Input: part model. Units: mm. Frame: model coordinates. A direction names the side the tool comes from. Give positions to 0.01 mm unless a question says otherwise; leave off trailing zeros. Loops run counter-clockwise (first coordinate to the right, second up) from the corner with the lowest first, then second, coordinate; pieces in that order, holes last. Notation, with made-up numbers: M -37.75,27.5 L -16.75,27.5 A21 cw -16.75,44.5 Z; hole C 27,85 d4. An arc over 180 degrees is marked long. Return JSON: item names as keys, results as strings. Group by question number.
```python
from build123d import *

# Parameters (mm, degrees)
F0_W      = 76.2
F0_H      = 76.2
F1_DEPTH  = 76.2
F3_D      = 25.4
F4_W      = 25.4
F4_H      = 25.4
F5_DEPTH  = 12.7
F6_R      = 12.7
F7_DEPTH  = 12.7
F8_R      = 12.7
F9_R      = 12.7
F10_SIZE  = 5.08
F11_SIZE  = 5.08
F12_R     = 5.08
F14_DEPTH = 7.62
F16_DEPTH = 7.62
F18_DEPTH = 7.62
F20_DEPTH = 7.62
F22_DEPTH = 7.62
F24_DEPTH = 7.62


with BuildPart() as f1:
    # F0 (on Front) → F1 (new body)
    with BuildSketch(Plane.XZ):
        with Locations((38.1, 38.1)):
            Rectangle(F0_W, F0_H)
    extrude(amount=F1_DEPTH)

    # F3 (through all)
    with Locations(Plane.XY.offset(76.2)):
        with Locations((37.350509, -33.948544)):
            Hole(F3_D / 2)

    # F4 (on face) → F5 (join)
    with BuildSketch(Plane.XZ.offset(76.2)):
        with Locations((38.1, 38.1)):
            Rectangle(F4_W, F4_H)
    extrude(amount=F5_DEPTH)

    # F6 (on face) → F7 (join)
    with BuildSketch(Plane.YZ.offset(76.2)):
        with Locations((-34.955569, 38.1)):
            Circle(F6_R)
    extrude(amount=F7_DEPTH)

    # F8
    f8_edges = [f1.edges().sort_by_distance(p)[0] for p in [
        (0, -38.1, 76.2),
    ]]
    fillet(f8_edges, radius=F8_R)

    # F9
    f9_edges = [f1.edges().sort_by_distance(p)[0] for p in [
        (76.2, -38.1, 76.2),
    ]]
    fillet(f9_edges, radius=F9_R)

    # F10
    f10_edges = [f1.edges().sort_by_distance(p)[0] for p in [
        (0, -76.2, 31.75),
    ]]
    chamfer(f10_edges, length=F10_SIZE)

    # F11
    f11_edges = [f1.edges().sort_by_distance(p)[0] for p in [
        (82.55, -22.255569, 38.1),
        (76.2, -47.655569, 38.1),
        (88.9, -47.655569, 38.1),
    ]]
    chamfer(f11_edges, length=F11_SIZE)

    # F12
    f12_edges = [f1.edges().sort_by_distance(p)[0] for p in [
        (38.1, -88.9, 50.8),
        (25.4, -88.9, 38.1),
        (38.1, -88.9, 25.4),
        (50.8, -88.9, 38.1),
    ]]
    fillet(f12_edges, radius=F12_R)

    # F13 (on face) → F14 (join)
    with BuildSketch(Plane(origin=(0, 0, 0), x_dir=(0, -1, 0), z_dir=(-1, 0, 0))):
        Polygon((25.23751, 33.285815), (31.410398, 33.285815), (35.259131, 38.111974), (33.885534, 44.130095), (28.323954, 46.808411), (22.762373, 44.130095), (21.388777, 38.111974), align=None)
    extrude(amount=F14_DEPTH)

    # F15 (on face) → F16 (join)
    with BuildSketch(Plane(origin=(0, 0, 0), x_dir=(0, -1, 0), z_dir=(-1, 0, 0))):
        Polygon((50.743747, 16.11791), (55.522759, 21.096045), (54.610361, 27.936243), (48.693608, 31.487695), (42.227936, 29.076085), (40.082127, 22.517406), (43.87202, 16.750475), align=None)
    extrude(amount=F16_DEPTH)

    # F17 (on face) → F18 (join)
    with BuildSketch(Plane(origin=(0, 0, 0), x_dir=(0, -1, 0), z_dir=(-1, 0, 0))):
        Polygon((57.059099, 37.974671), (63.266012, 45.136495), (60.167147, 54.092752), (50.861369, 55.887184), (44.654456, 48.72536), (47.753321, 39.769104), align=None)
    extrude(amount=F18_DEPTH)

    # F19 (on face) → F20 (join)
    with BuildSketch(Plane(origin=(0, 0, 0), x_dir=(0, -1, 0), z_dir=(-1, 0, 0))):
        Polygon((17.242883, 6.356385), (22.038512, 11.837104), (21.55408, 19.10358), (16.07336, 23.89921), (8.806884, 23.414778), (4.011255, 17.934058), (4.495687, 10.667582), (9.976407, 5.871953), align=None)
    extrude(amount=F20_DEPTH)

    # F21 (on face) → F22 (join)
    with BuildSketch(Plane(origin=(0, 0, 0), x_dir=(0, -1, 0), z_dir=(-1, 0, 0))):
        Polygon((11.161887, 45.752136), (17.368809, 51.004144), (15.923897, 59.0055), (8.272064, 61.754847), (2.065142, 56.502839), (3.510054, 48.501483), align=None)
    extrude(amount=F22_DEPTH)

    # F23 (on face) → F24 (join)
    with BuildSketch(Plane(origin=(0, 0, 0), x_dir=(0, -1, 0), z_dir=(-1, 0, 0))):
        Polygon((58.197337, 4.173143), (61.300796, 8.231508), (59.337879, 12.948366), (54.271501, 13.606857), (51.168042, 9.548492), (53.13096, 4.831635), align=None)
    extrude(amount=F24_DEPTH)


solid = f1.part
```
Item 1: Material intervals for line 1 (Y direction, x = 37.5, z = 15); line 2 (X direction, y = -69, z = 54.5); line 3 (X direction, y = -49, z = 17), sorted ascending. Write a range as from..to.
Item 2: Reachability of faces 1 (the face through (-3.757, -55.579, 54.977)), 2 (the face through (-3.757, -52.341, 38.884)), 3 (the face through (-3.76, -41.17, 25.84)), 4 (the face through (-3.757, -56.84, 13.273)) from +Z, -Z, +X, -X, +Y, -Y: full face, straight path, thin tool, end or side. Return the list, or none.
Item 3: Section A-A, the plane x = 32. Return loops of the section in (y, z), then the cut area to 3 significant figures.
Item 4: Pull-direction query (Y, two-part tool) for faces 5 (the face through (73.62, -73.7, 32.19)), 6 (the face through (-3.757, -16.656, 54.949)), 7 (the face through (26, -27, 76.2)), 8 (the face through (-3.76, -12.49, 23.66)); classes: pulls with the +Y half, pulls with the -Y half, needs draft (parallel to the pull), parting line crosses it, or undercut.
Item 5: First-contact query: pin 1 Ø8.5 at (y, z) = (-78.5, 40.5) entering from +X; pin 2 Ø3 at (x, z) = (74.5, 26.5) entering from -Y; pin 3 Ø5 at (x, y) = (-5, -29) entering from -Z. Flat tips, straight axial feed; report the tip coordinate or a pass-through.
Item 6: Section B-B, the plane y = -79.5. Return loops of the section in (x, z), then the cut area to 3 significant figures.
Item 7: Section C-C, the plane x = 58.5. Return loops of the section in (y, z).
Answer below:
{
 "1": {"line 1": "-76.2..-46.65, -21.25..0", "line 2": "0..76.2", "line 3": "-7.62..76.2"},
 "2": {"face 1": "+Z, -X, -Y", "face 2": "-X", "face 3": "+Z, -X", "face 4": "-X, -Y"},
 "3": {"outline": "M -88.9,30.48 A5.08 ccw -83.82,25.4 L -76.2,25.4 L -76.2,0 L -45.47,0 L -45.47,76.2 L -71.12,76.2 L -76.2,71.12 L -76.2,50.8 L -83.82,50.8 A5.08 ccw -88.9,45.72 Z; M -22.43,0 L 0,0 L 0,76.2 L -22.43,76.2 Z", "area": "4,350 mm^2"},
 "4": {"face 5": "pulls with the -Y half", "face 6": "undercut", "face 7": "needs draft", "face 8": "pulls with the +Y half"},
 "5": {"pin 1": "x = 73.07", "pin 2": "y = -74.32", "pin 3": "z = 33.29"},
 "6": {"outline": "M 25.4,25.4 L 50.8,25.4 L 50.8,50.8 L 25.4,50.8 Z", "area": "645 mm^2"},
 "7": {"outline": "M -76.2,0 L 0,0 L 0,76.2 L -71.12,76.2 L -76.2,71.12 Z"}
}
